Drawing for the job (mm, zero at the part's lowest x, y, z). A direction names the side the tool comes from. Give positions to 0.01 mm unless a question says otherwise; leave off trailing zeros. Order: outer loops, then holes, each group sorted by start corner. A loop starts at its lowest first (then second) coordinate and runs counter-clockwise, first axis right, second up. Notation, with made-up numbers: (-23, 82) - (29, 82) arc R16 cw to (29, 94) - close; hole circle Ø11 at (-12.5, 18). An arc over 180 degrees is marked (long way). Use CSV: the item, a comma, the result in double quotes. Start each with the question number.
(1) Tool access for the marked faces 1 and 2: list every direction of +Z, -Z, +X, -X, +Y, -Y with a clear straight run to the whole face (end or side of a thin tool).
(2) Band-saw the part on C-C, the plane x = 3.25. Give the cut face in (y, z) (1 decimal), then the cut area to 3 significant figures.
(3) Band-saw the part on A-A, the plane z = 56. Give the cut face in (x, y).
(4) Band-saw the part on B-B, the plane z = 23.5. Give the cut face in (x, y).
(5) Band-saw the part on D-D, the plane y = 5.5. Give the cut face in (x, z) (1 decimal).
(6) Drop flat-ended pins along their axis: pin 1 Ø4 at (y, z) = (7.5, 8.5) entering from -X; pin 2 Ø2 at (x, y) = (4, 4.62) entering from +Z; pin 3 Ø1.5 at (x, y) = (6, 1.5) entering from -Z. Give the stop position or say it passes through.
(7) Probe L1, parallel to Y at x = 4, z = 57.5; L2, parallel to X at y = 4.5, z = 54 (1 decimal); L3, parallel to Z at x = 2.25, y = 6.75. List the from-to ranges inside material, lowest first.
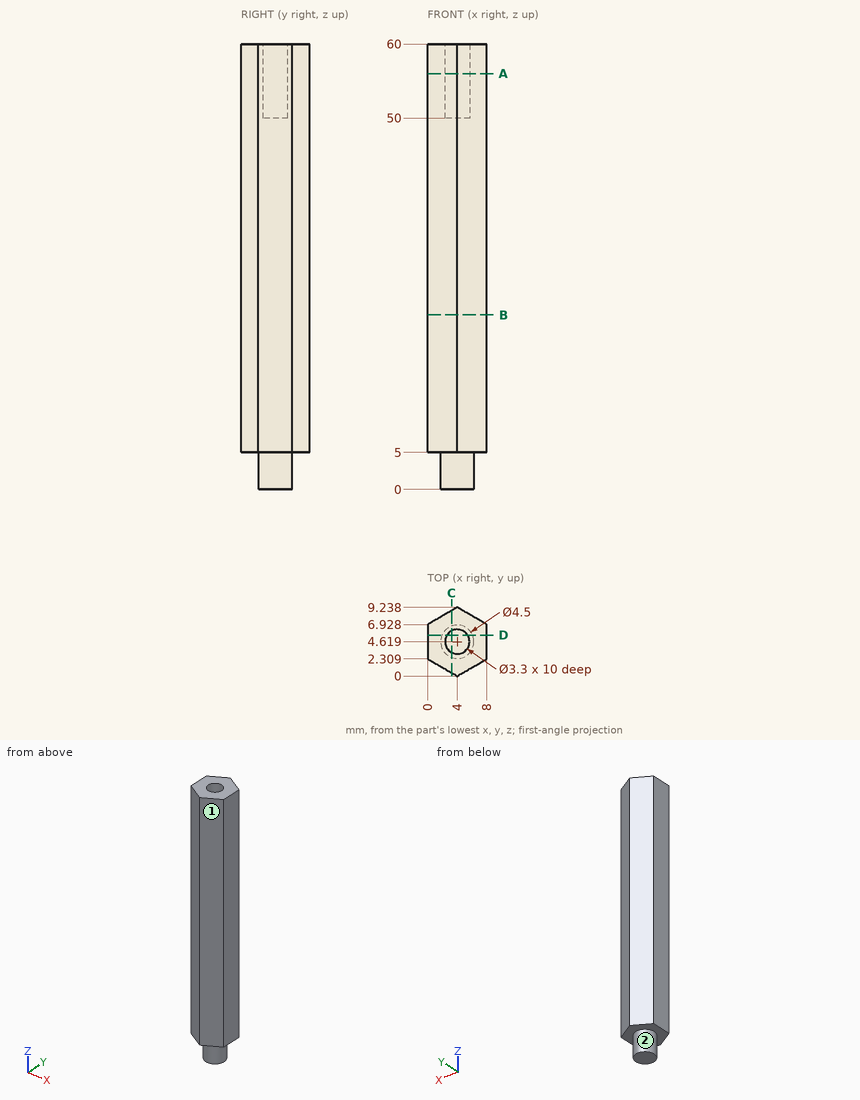
Answer block:
1,face 1,"+Z, -Z, +X, -Y"
1,face 2,"-Z"
2,outline,"(0.4, 5) - (2.5, 5) - (2.5, 0) - (6.7, 0) - (6.7, 5) - (8.8, 5) - (8.8, 60) - (6.1, 60) - (6.1, 50) - (3.1, 50) - (3.1, 60) - (0.4, 60) - close"
2,area,"452 mm2"
3,outline,"(0, 2.31) - (4, 0) - (8, 2.31) - (8, 6.93) - (4, 9.24) - (0, 6.93) - close; hole circle Ø3.3 at (4, 4.62)"
4,outline,"(0, 2.31) - (4, 0) - (8, 2.31) - (8, 6.93) - (4, 9.24) - (0, 6.93) - close"
5,outline,"(0, 5) - (1.9, 5) - (1.9, 0) - (6.1, 0) - (6.1, 5) - (8, 5) - (8, 60) - (5.4, 60) - (5.4, 50) - (2.6, 50) - (2.6, 60) - (0, 60) - close"
6,pin 1,"stops at x = 0"
6,pin 2,"stops at z = 50"
6,pin 3,"stops at z = 5"
7,L1,"y = 0 to 2.97, 6.27 to 9.24"
7,L2,"x = 0 to 2.4, 5.6 to 8"
7,L3,"z = 5 to 60"
